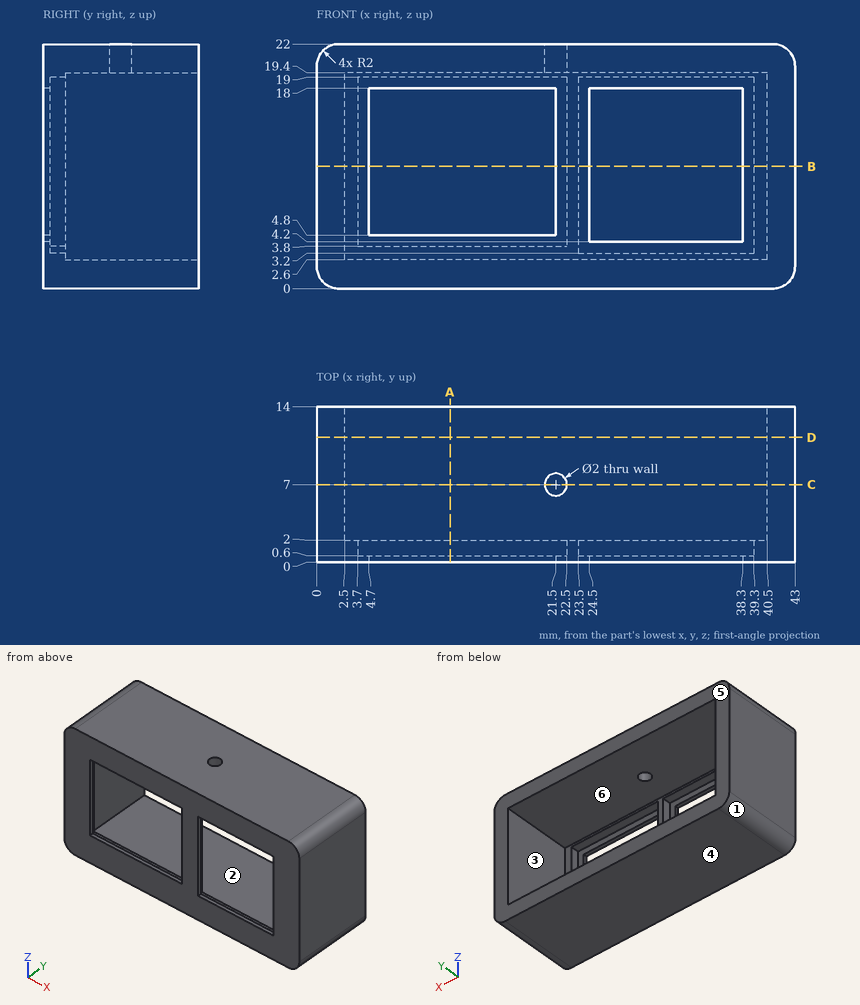
Study the drawing (mm; zero at the part's minimum x, y, z) and answer. A direction names the side the tool comes from. Round coordinates to 2 decimals unless told otherwise and drop trailing zeros. Write each loop counter-clockwise with the first axis right and the second up, starting at its lowest first coordinate (ties: lowest second). Pieces come first, ordered by that corner, then holes. Notation, with made-up numbers: (-20.75, -8) - (26.25, -8) arc R23 cw to (26.25, 31) - close; hole circle Ø5 at (36, 0). An arc over 180 degrees is marked (long way). Use a Markdown table: item, result. Add a question column.
1. The part is cut by section D-D (y = 11.25). Write down the section's boundary in (x, z), and give its area (3 significant figures).
2. Flat-ended cylindrical pins translate along their axes: P1, Ø6, axis at x = 22, z = 9.5, coming from the +Y side; P2, Ø8.5, axis at x = 14.5, z = 12.5, coming from the +Y side. Find the tip coordinate at first contact, or state that the pin passes through.
3. For a pull along Z with two mould halves and no side action, classify the marked faces 3, 4, 5 and 6 as +Z half, -Z half, draft (parallel to the pull), parting line (faces both ways), or undercut.
4. A tool of negligible diameter and unlimited length cuts with its end or side. For the marked faces 1 and 2, from which of +Z, -Z, +X, -X, +Y, -Y can it reach the whole face along a straight path? Write none if from no direction.
5. Consider line 1 (X direction, y = 1.75, z = 5.25); line 2 (Z direction, x = 9, y = 9); line 3 (X direction, y = 4.75, z = 10.75). Determine where each line is inside the solid, lowest interval first.
6. The part is cut by section A-A (x = 12). Write down the section's boundary in (y, z), and give its area (3 significant figures).
7. The part is cut by section B-B (z = 11). Write down the section's boundary in (x, y).
8. The part is cut by section C-C (y = 7). Write down the section's boundary in (x, z).
Reported:
| question | item | result |
|---|---|---|
| 1 | outline | (0, 2) arc R2 ccw to (2, 0) - (41, 0) arc R2 ccw to (43, 2) - (43, 20) arc R2 ccw to (41, 22) - (2, 22) arc R2 ccw to (0, 20) - close; hole (2.5, 2.6) - (40.5, 2.6) - (40.5, 19.4) - (2.5, 19.4) - close |
| 1 | area | 304 mm^2 |
| 2 | P1 | y = 2 |
| 2 | P2 | through |
| 3 | face 3 | undercut |
| 3 | face 4 | -Z half |
| 3 | face 5 | draft |
| 3 | face 6 | undercut |
| 4 | face 1 | -Z, -X, +Y, -Y |
| 4 | face 2 | +Y |
| 5 | line 1 | 0 to 3.7, 22.5 to 23.5, 39.3 to 43 |
| 5 | line 2 | 0 to 2.6, 19.4 to 22 |
| 5 | line 3 | 0 to 2.5, 40.5 to 43 |
| 6 | outline | (0, 0) - (14, 0) - (14, 2.6) - (2, 2.6) - (2, 3.8) - (0.6, 3.8) - (0.6, 4.8) - (0, 4.8) - close; (0, 18) - (0.6, 18) - (0.6, 19) - (2, 19) - (2, 19.4) - (14, 19.4) - (14, 22) - (0, 22) - close |
| 6 | area | 77.2 mm^2 |
| 7 | outline | (0, 0) - (4.7, 0) - (4.7, 0.6) - (3.7, 0.6) - (3.7, 2) - (2.5, 2) - (2.5, 14) - (0, 14) - close; (21.5, 0) - (24.5, 0) - (24.5, 0.6) - (23.5, 0.6) - (23.5, 2) - (22.5, 2) - (22.5, 0.6) - (21.5, 0.6) - close; (38.3, 0) - (43, 0) - (43, 14) - (40.5, 14) - (40.5, 2) - (39.3, 2) - (39.3, 0.6) - (38.3, 0.6) - close |
| 8 | outline | (0, 2) arc R2 ccw to (2, 0) - (41, 0) arc R2 ccw to (43, 2) - (43, 20) arc R2 ccw to (41, 22) - (22.5, 22) - (22.5, 19.4) - (40.5, 19.4) - (40.5, 2.6) - (2.5, 2.6) - (2.5, 19.4) - (20.5, 19.4) - (20.5, 22) - (2, 22) arc R2 ccw to (0, 20) - close |
